Check sheet for the drawn part. Datum: minimum x, y, z corner. Units: mm. A direction names the side the tool comes from. Give positions to 0.01 mm unless a question says otherwise; leave off trailing zeros. Answer as a JSON object with one key per item and string values. Group by question number.
Item 1: Scan lines: line 1 along Y through (x, z) = (88, 38) (1 decimal); line 2 along X through (y, z) = (88.9, 37) (1 decimal); line 3 along X through (y, z) = (71, 41.5) (1 decimal). Record each from-to range of solid material in increasing order. Write a range as [from, to].
Item 2: Tool access check on the marked faces 4, 5 and 6. Record the directions out of +Z, -Z, +X, -X, +Y, -Y that give a thin tool (end or side, any length) a straight path to the whole face; none if there is none.
Item 3: Draft check along X on the marked faces 1, 2 and 3. Enter one of: +X half, -X half, draft (parallel to the pull), parting line (faces both ways), or undercut.
Item 4: Go/stop test with flat-tipped pins: pin 1 (1 mm diameter, centred on x = 133, y = 77, fed in from -Z) (3 decimals); pin 2 (3 mm diameter, centred on x = 28, z = 20.5, fed in from +Y); pin 3 (4 mm diameter, centred on y = 130, z = 30, fed in from -X); pin 4 (1.9 mm diameter, centred on x = 88.5, z = 14.5, fed in from -Y). Record where each tip stops, or that it passes through.
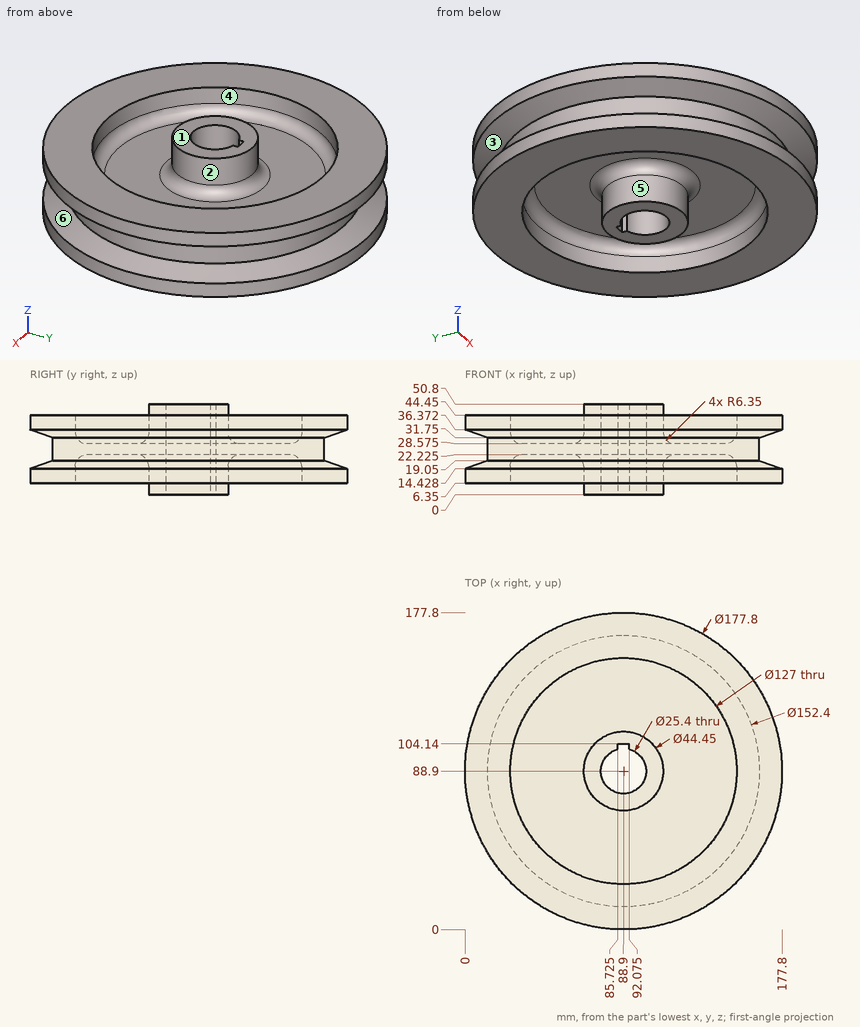
Geometry check:
{
 "1": {"line 1": "[0, 25.4], [66.7, 76.2], [104.1, 111.1], [152.4, 177.8]", "line 2": "[0, 25.4], [66.7, 76.2], [101.6, 111.1], [152.4, 177.8]", "line 3": "[1.8, 28], [75.7, 102.1], [149.8, 176]"},
 "2": {"face 4": "+Z", "face 5": "-Z", "face 6": "none"},
 "3": {"face 1": "draft", "face 2": "undercut", "face 3": "parting line"},
 "4": {"pin 1": "z = 22.225", "pin 2": "y = 136.63", "pin 3": "x = 23.5", "pin 4": "y = 0"}
}
